from build123d import *

# Parameters (mm, degrees)
SKETCH1_W                = 160
SKETCH1_H                = 436
BOSS_EXTRUDE1_DEPTH      = 12.7
CUT_EXTRUDE1_DEPTH       = 366.47051465
CIRPATTERN1_COUNT        = 3
CIRPATTERN1_ANGLE        = 102.52
CUT_EXTRUDE2_DEPTH       = 366.47051465
CIRPATTERN2_COUNT        = 2
CIRPATTERN2_ANGLE        = 51.26
F_5_0_5_DIAMETER_HOLE1_D = 5
CUT_EXTRUDE3_DEPTH       = 366.47051465


with BuildPart() as part:
    # Sketch1 → Boss-Extrude1 (new body)
    with BuildSketch(Plane.XY):
        with Locations((74.181489842, 113.112481294)):
            Rectangle(SKETCH1_W, SKETCH1_H)
    extrude(amount=BOSS_EXTRUDE1_DEPTH)

    # Sketch3 → Cut-Extrude1 (cut, through all)
    with BuildSketch(Plane(origin=(0, 0, 0), x_dir=(-1, 0, 0), z_dir=(0, 0, -1))):
        with BuildLine():
            Line((-59.468207995, 200.039680409), (-47.878421887, 206.962603057))
            ThreePointArc((-47.878421887, 206.962603057), (-47.604309032, 207.331039293), (-47.671005734, 207.785390113))
            Line((-47.671005734, 207.785390113), (-49.508913494, 210.862263699))
            ThreePointArc((-49.508913494, 210.862263699), (-49.87734973, 211.136376554), (-50.33170055, 211.069679852))
            Line((-50.33170055, 211.069679852), (-61.921486657, 204.146757205))
            ThreePointArc((-61.921486657, 204.146757205), (-62.195599513, 203.778320969), (-62.128902811, 203.323970149))
            Line((-62.128902811, 203.323970149), (-60.29099505, 200.247096563))
            ThreePointArc((-60.29099505, 200.247096563), (-59.922558815, 199.972983708), (-59.468207995, 200.039680409))
        make_face()
        with BuildLine():
            Line((-94.041533827, 186.486629291), (-85.165935337, 196.658834137))
            ThreePointArc((-85.165935337, 196.658834137), (-85.019418624, 197.094053588), (-85.223562287, 197.505403175))
            Line((-85.223562287, 197.505403175), (-87.924094299, 199.861710211))
            ThreePointArc((-87.924094299, 199.861710211), (-88.35931375, 200.008226924), (-88.770663336, 199.804083262))
            Line((-88.770663336, 199.804083262), (-97.646261826, 189.631878415))
            ThreePointArc((-97.646261826, 189.631878415), (-97.79277854, 189.196658964), (-97.588634877, 188.785309377))
            Line((-97.588634877, 188.785309377), (-94.888102864, 186.429002341))
            ThreePointArc((-94.888102864, 186.429002341), (-94.452883414, 186.282485628), (-94.041533827, 186.486629291))
        make_face()
    cut_extrude1 = extrude(amount=-CUT_EXTRUDE1_DEPTH, mode=Mode.SUBTRACT)

    # CirPattern1: Cut-Extrude1 ×3 about axis
    cirpattern1_axis = Axis((-0.318510158, 113.112481294, 0), (0, 0, -1))
    for i in range(1, CIRPATTERN1_COUNT):
        add(cut_extrude1.rotate(cirpattern1_axis, i * CIRPATTERN1_ANGLE / (CIRPATTERN1_COUNT - 1)), mode=Mode.SUBTRACT)

    # Sketch4 → Cut-Extrude2 (cut, through all)
    with BuildSketch(Plane(origin=(0, 0, 0), x_dir=(-1, 0, 0), z_dir=(0, 0, -1))):
        with BuildLine():
            Line((-124.50767277, 163.337281817), (-121.260766753, 161.81983089))
            ThreePointArc((-121.260766753, 161.81983089), (-120.80200107, 161.799406266), (-120.463162354, 162.109360202))
            Line((-120.463162354, 162.109360202), (-114.747317623, 174.339614451))
            ThreePointArc((-114.747317623, 174.339614451), (-114.726892999, 174.798380135), (-115.036846934, 175.13721885))
            Line((-115.036846934, 175.13721885), (-118.283752952, 176.654669778))
            ThreePointArc((-118.283752952, 176.654669778), (-118.742518635, 176.675094401), (-119.081357351, 176.365140466))
            Line((-119.081357351, 176.365140466), (-124.797202082, 164.134886216))
            ThreePointArc((-124.797202082, 164.134886216), (-124.817626706, 163.676120533), (-124.50767277, 163.337281817))
        make_face()
    cut_extrude2 = extrude(amount=-CUT_EXTRUDE2_DEPTH, mode=Mode.SUBTRACT)

    # CirPattern2: Cut-Extrude2 ×2 about axis
    cirpattern2_axis = Axis((-0.318510158, 113.112481294, 0), (0, 0, -1))
    for i in range(1, CIRPATTERN2_COUNT):
        add(cut_extrude2.rotate(cirpattern2_axis, i * CIRPATTERN2_ANGLE / (CIRPATTERN2_COUNT - 1)), mode=Mode.SUBTRACT)

    # Ø5.0 (5) Diameter Hole1 (through all)
    with Locations(Plane(origin=(0, 0, 0), x_dir=(-1, 0, 0), z_dir=(0, 0, -1))):
        with Locations((-142.931489842, 113.112481294)):
            f_5_0_5_diameter_hole1 = Hole(F_5_0_5_DIAMETER_HOLE1_D / 2)

    # Sketch-Pattern9: Ø5.0 (5) Diameter Hole1 at 3 more places
    with Locations((-42.5, 0, 0), (-125.75, 109.358642, 0), (-125.75, -109.358642, 0)):
        add(f_5_0_5_diameter_hole1, mode=Mode.SUBTRACT)

    # Sketch9 → Cut-Extrude3 (cut, through all)
    with BuildSketch(Plane(origin=(0, 0, 0), x_dir=(-1, 0, 0), z_dir=(0, 0, -1))):
        with BuildLine():
            Line((5.818510158, 276.362481294), (-3.931489842, 276.362481294))
            ThreePointArc((-3.931489842, 276.362481294), (-4.638596623, 276.069588075), (-4.931489842, 275.362481294))
            Line((-4.931489842, 275.362481294), (-4.931489842, 225.362481294))
            ThreePointArc((-4.931489842, 225.362481294), (-4.638596623, 224.655374512), (-3.931489842, 224.362481294))
            Line((-3.931489842, 224.362481294), (5.818510158, 224.362481294))
            Line((5.818510158, 224.362481294), (5.818510158, 276.362481294))
        make_face()
        with BuildLine():
            Line((-32.181489842, 331.112481294), (-0.181489842, 331.112481294))
            Line((-0.181489842, 331.112481294), (-0.181489842, 321.362481294))
            ThreePointArc((-0.181489842, 321.362481294), (-0.474383061, 320.655374512), (-1.181489842, 320.362481294))
            Line((-1.181489842, 320.362481294), (-31.181489842, 320.362481294))
            ThreePointArc((-31.181489842, 320.362481294), (-31.888596623, 320.655374512), (-32.181489842, 321.362481294))
            Line((-32.181489842, 321.362481294), (-32.181489842, 331.112481294))
        make_face()
    cut_extrude3 = extrude(amount=-CUT_EXTRUDE3_DEPTH, mode=Mode.SUBTRACT)

    # Mirror1: Cut-Extrude3 across plane
    add(cut_extrude3.mirror(Plane.ZX.offset(113.112481294)), mode=Mode.SUBTRACT)


solid = part.part
Model file for the job. Use its own axes, mm. A direction names the side the tool comes from. Coordinates: 2 decimals unless noted, no trailing zeros. Order: outer loops, then holes, each group sorted by start corner. A loop starts at its lowest first (then second) coordinate and runs counter-clockwise, first axis right, second up. Notation, with made-up numbers: M 39,87 L 54,87 A20 cw 54,106 Z; hole C 75,-18.75 d1. An arc over 180 degrees is marked long. Return JSON: item names as keys, results as strings.
1. Tool access for faces 1 (the face through (32.181, 326, 6)), 2 (the face through (32.181, -100, 6)), 3 (the face through (76.15, 40.74, 6.26)): list every direction of +Z, -Z, +X, -X, +Y, -Y with a clear straight run to the whole face (end or side of a thin tool).
Ans:
{"face 1": "+Z, -Z, +Y", "face 2": "+Z, -Z, -Y", "face 3": "+Z, -Z"}
2. Saw through at B-B (x = 24.5). Give the cut face in (y, z).
Ans:
{"outline": "M -94.14,0 L 320.36,0 L 320.36,12.7 L -94.14,12.7 Z"}
3. Drill centre lines: probe 1 along Y at (x, z) = (2, 10.25); probe 2 along Y at (x, z) = (56, 6); probe 3 along X at (y, z) = (111.5, 7.5). Where is each one in solid material? Low to high.
Ans:
{"probe 1": "-94.14 to -50.14, 1.86 to 224.36, 276.36 to 320.36", "probe 2": "-104.89 to 2.45, 7.89 to 202.11, 207.68 to 331.11", "probe 3": "-5.82 to 98.52, 102.34 to 141.02, 144.84 to 154.18"}
4. Saw through at C-C (z = 3.5). Give the number of separate pieces and of enclosed holes in the cut face, and give its area (3 significant figures).
Ans:
{"separate pieces": "1", "enclosed holes": "12", "area": "67,300 mm^2"}
5. Flat gauge pins, fed straight in: pin 1 (6.5 mm diameter, centred on x = 16, z = 3.5, fed in from -Y); pin 2 (4.5 mm diameter, centred on x = 100.43, y = 113.11, fed in from -Z); pin 3 (5 mm diameter, centred on x = 1.5, z = 9.5, fed in from +Y); pin 4 (6.5 mm diameter, centred on y = 262.5, z = 6.5, fed in from -X). Where does each tip first touch, or does it go through?
Ans:
{"pin 1": "y = -94.14", "pin 2": "through", "pin 3": "y = 331.11", "pin 4": "x = 4.93"}
6. Pull direction Y, two halves, no side cores. Call faces 4 (the face through (92, -104.888, 6)), 5 (the face through (121.878, 91.323, 6.261)), 6 (the face through (59.15, 4.16, 6.26)), 7 (the face through (154.181, 110, 6)): +Y half, -Y half, draft (parallel to the pull), parting line (faces both ways), or undercut.
Ans:
{"face 4": "-Y half", "face 5": "undercut", "face 6": "undercut", "face 7": "draft"}
7. Saw through at A-A (y = -13.5). Give the cut face in (x, z), and give its area (3 significant figures).
Ans:
{"outline": "M 4.93,0 L 154.18,0 L 154.18,12.7 L 4.93,12.7 Z", "area": "1,900 mm^2"}
